Could you check a few things on this model? Use its own coordinates, in mm. Face numbers are marked on the shaded views. A direction names the side the tool comes from. Give positions to 0.01 mm unless a question says otherwise; leave off trailing zeros. Loops run counter-clockwise (first coordinate to the right, second up) from the corner with the lowest first, then second, coordinate; pieces in that order, holes last. Notation, with made-up numbers: M -39.75,60 L 16.25,60 A29 cw 16.25,97 Z; hole C -32.75,69.5 d9. An arc over 180 degrees is marked long. Return JSON: item names as keys, results as strings. Group by question number.
1. If we mould it in two halves opening along Z, with no side actions, what happens to the marked faces 4, 5 and 6? For each: +Z half, -Z half, draft (parallel to the pull), parting line (faces both ways), or undercut.
2. For the marked faces 1, 2 and 3, which set-ups out of +Z, -Z, +X, -X, +Y, -Y let a thin tool reach every point of the face, with its end or its side?
3. For pin 1 (5.5 mm diameter, centred on x = 8.95, y = 27.36, fed in from +Z) (3 decimals); pin 2 (1 mm diameter, centred on y = 8.5, z = 20.5, fed in from +X) (3 decimals); pin 3 (2.5 mm diameter, centred on x = 38.1, z = 12.7, fed in from -Y); pin 4 (5 mm diameter, centred on x = 3.5, z = 16.5, fed in from -Y), each with a flat end and sliding along its axis, tell me the tip position at first contact or that it passes through.
4. Please list where these lines run through material, in increasing order: line 1 (X direction, y = 0.75, z = 12.7); line 2 (X direction, y = 44, z = 2); line 3 (X direction, y = 36, z = 20.5) (3 decimals).
5. If we section it at A-A (y = 38.1): Write out the boundary of the cut face in (x, z) (3 decimals), plus the area to 3 significant figures.
6. If we section it at C-C (x = 50.8): Write out the boundary of the cut face in (y, z) (3 decimals), plus the area to 3 significant figures.
7. If we section it at B-B (z = 9.5): Write out the boundary of the cut face in (x, y) (3 decimals), plus the area to 3 significant figures.
```python
from build123d import *

# Parameters (mm, degrees)
BOSS_EXTRUDE1_DEPTH        = 3.175
SKETCH2_W                  = 6.477
SKETCH2_H                  = 6.477
CUT_EXTRUDE1_DEPTH         = 4.175
SKETCH3_W                  = 63.246
SKETCH3_H                  = 3.175
BOSS_EXTRUDE2_DEPTH        = 22.225
SKETCH4_W                  = 3.175
SKETCH4_H                  = 63.246
BOSS_EXTRUDE3_DEPTH        = 22.225
M6_5_CLEARANCE_HOLE1_D     = 7.4422
M6_5_CLEARANCE_HOLE1_DEPTH = 25.400025
M25_CLEARANCE_HOLE1_D      = 28.575
M25_CLEARANCE_HOLE1_DEPTH  = 25.400025
HOLE1_D                    = 4.9784
HOLE1_DEPTH                = 25.400025
M3_5_CLEARANCE_HOLE1_D     = 4.1402
M3_5_CLEARANCE_HOLE1_DEPTH = 25.400025
M3_5_CLEARANCE_HOLE2_D     = 4.1402
M3_5_CLEARANCE_HOLE2_DEPTH = 3.175
M3_5_CLEARANCE_HOLE3_D     = 4.1402
M3_5_CLEARANCE_HOLE3_DEPTH = 3.175
CHAMFER1_SIZE              = 2.159
FILLET1_R                  = 1.2192
FILLET2_R                  = 2.0701
FILLET3_R                  = 4.3942


with BuildPart() as part:
    # Sketch1 → Boss-Extrude1 (new body)
    with BuildSketch(Plane(origin=(0, 0, 0), x_dir=(-1, 0, 0), z_dir=(0, 0, -1))):
        Polygon((-69.723, 0), (0, 0), (0, 69.723), (-16.428128061, 69.723), (-69.723, 16.428128061), align=None)
    extrude(amount=-BOSS_EXTRUDE1_DEPTH)

    # Sketch2 → Cut-Extrude1 (cut, through all)
    with BuildSketch(Plane(origin=(0, 0, 0), x_dir=(-1, 0, 0), z_dir=(0, 0, -1))):
        with Locations((-3.2385, 3.2385)):
            Rectangle(SKETCH2_W, SKETCH2_H)
    extrude(amount=-CUT_EXTRUDE1_DEPTH, mode=Mode.SUBTRACT)

    # Sketch3 → Boss-Extrude2 (add)
    with BuildSketch(Plane.XY.offset(3.175)):
        with Locations((38.1, 1.5875)):
            Rectangle(SKETCH3_W, SKETCH3_H)
    extrude(amount=BOSS_EXTRUDE2_DEPTH)

    # Sketch4 → Boss-Extrude3 (add)
    with BuildSketch(Plane.XY.offset(3.175)):
        with Locations((1.5875, 38.1)):
            Rectangle(SKETCH4_W, SKETCH4_H)
    extrude(amount=BOSS_EXTRUDE3_DEPTH)

    # M6.5 Clearance Hole1
    with Locations(Plane(origin=(0, 0, 0), x_dir=(-1, 0, 0), z_dir=(0, 0, -1))):
        with Locations((-9.85939269, 9.85939269)):
            Hole(M6_5_CLEARANCE_HOLE1_D / 2, depth=M6_5_CLEARANCE_HOLE1_DEPTH)

    # M25 Clearance Hole1
    with Locations(Plane(origin=(0, 0, 0), x_dir=(-1, 0, 0), z_dir=(0, 0, -1))):
        with Locations((-27.360115818, 27.360115818)):
            Hole(M25_CLEARANCE_HOLE1_D / 2, depth=M25_CLEARANCE_HOLE1_DEPTH)

    # Hole1
    with Locations(Plane(origin=(0, 0, 0), x_dir=(-1, 0, 0), z_dir=(0, 0, -1))):
        with Locations((-9.399603576, 45.320628061), (-45.320628061, 9.399603576)):
            Hole(HOLE1_D / 2, depth=HOLE1_DEPTH)

    # M3.5 Clearance Hole1
    with Locations(Plane(origin=(0, 0, 0), x_dir=(-1, 0, 0), z_dir=(0, 0, -1))):
        with Locations((-45.775115818, 27.360115818), (-8.945115818, 27.360115818), (-27.360115818, 45.775115818), (-27.360115818, 8.945115818)):
            Hole(M3_5_CLEARANCE_HOLE1_D / 2, depth=M3_5_CLEARANCE_HOLE1_DEPTH)

    # M3.5 Clearance Hole2
    with Locations(Plane(origin=(3.175, 0, 0), x_dir=(0, 0, -1), z_dir=(1, 0, 0))):
        with Locations((-12.7, 63.5), (-12.7, 50.8), (-12.7, 38.1), (-12.7, 25.4), (-12.7, 12.7)):
            Hole(M3_5_CLEARANCE_HOLE2_D / 2, depth=M3_5_CLEARANCE_HOLE2_DEPTH)

    # M3.5 Clearance Hole3
    with Locations(Plane(origin=(0, 3.175, 0), x_dir=(1, 0, 0), z_dir=(0, 1, 0))):
        with Locations((63.5, -12.7), (50.8, -12.7), (38.1, -12.7), (25.4, -12.7), (12.7, -12.7)):
            Hole(M3_5_CLEARANCE_HOLE3_D / 2, depth=M3_5_CLEARANCE_HOLE3_DEPTH)

    # Chamfer1
    chamfer1_edges = [part.edges().sort_by_distance(p)[0] for p in [
        (1.5875, 6.477, 25.4),
        (1.5875, 69.723, 25.4),
        (6.477, 1.5875, 25.4),
        (69.723, 1.5875, 25.4),
    ]]
    chamfer(chamfer1_edges, length=CHAMFER1_SIZE)

    # Fillet1
    fillet1_edges = [part.edges().sort_by_distance(p)[0] for p in [
        (38.1, 3.175, 3.175),
        (3.175, 38.1, 3.175),
    ]]
    fillet(fillet1_edges, radius=FILLET1_R)

    # Fillet2
    fillet2_edges = [part.edges().sort_by_distance(p)[0] for p in [
        (6.477, 6.477, 1.5875),
    ]]
    fillet(fillet2_edges, radius=FILLET2_R)

    # Fillet3
    fillet3_edges = [part.edges().sort_by_distance(p)[0] for p in [
        (0, 38.1, 0),
        (38.1, 0, 0),
    ]]
    fillet(fillet3_edges, radius=FILLET3_R)


solid = part.part
```
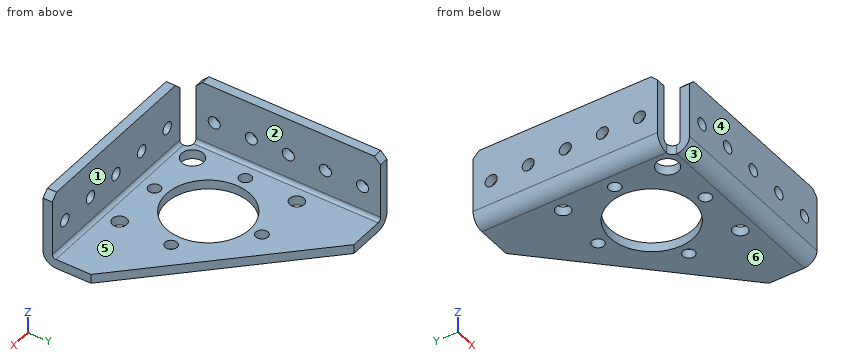
Answer:
{
 "1": {"face 4": "draft", "face 5": "+Z half", "face 6": "-Z half"},
 "2": {"face 1": "+Z, +X, -X, +Y", "face 2": "+Z, +X, +Y, -Y", "face 3": "-Z, +X, -X, -Y"},
 "3": {"pin 1": "stops at z = 3.175", "pin 2": "stops at x = 3.175", "pin 3": "passes through", "pin 4": "stops at y = 6.48"},
 "4": {"line 1": "x = 6.48 to 10.63, 14.77 to 23.33, 27.47 to 36.03, 40.17 to 48.73, 52.87 to 61.43, 65.57 to 69.72", "line 2": "x = 0.71 to 7.29, 11.51 to 26.3, 28.43 to 42.15", "line 3": "x = 0 to 3.175"},
 "5": {"outline": "M 0,4.394 A4.394 ccw 4.394,0 L 17.937,0 L 17.937,3.175 L 4.394,3.175 A1.219 cw 3.175,4.394 L 3.175,10.63 L 0,10.63 Z; M 0,14.77 L 3.175,14.77 L 3.175,25.4 L 0,25.4 Z; M 36.783,0 L 48.051,0 L 48.051,3.175 L 36.783,3.175 Z", "area": "146 mm²"},
 "6": {"outline": "M 0,4.394 A4.394 ccw 4.394,0 L 35.351,0 L 35.351,3.175 L 4.394,3.175 A1.219 cw 3.175,4.394 L 3.175,10.63 L 0,10.63 Z; M 0,14.77 L 3.175,14.77 L 3.175,25.4 L 0,25.4 Z", "area": "166 mm²"},
 "7": {"outline": "M 0,6.477 L 3.175,6.477 L 3.175,69.723 L 0,69.723 Z; M 6.477,0 L 69.723,0 L 69.723,3.175 L 6.477,3.175 Z", "area": "402 mm²"}
}
